Autodesk Inventor part; units mm, degrees
ref_plane "YZ Plane" through (0, 0, 0) normal (1, 0, 0) x (0, 1, 0)
ref_plane "XZ Plane" through (0, 0, 0) normal (0, 1, 0) x (-1, 0, 0)
ref_plane "XY Plane" through (0, 0, 0) normal (0, 0, 1) x (1, 0, 0)
sketch "Boceto1" plane through (0, 0, 0) normal (0, 1, 0) x (-1, 0, 0)
  circle A0 centre (0, 0) radius 0.99
  dimension "d0" = 1.98
extrude "Extrusión1" add sketch "Boceto1" along normal mid plane 4
sketch "Boceto2" plane through (0, 2, 0) normal (0, 1, 0) x (1, 0, 0)
  circle A0 centre (0, 0) radius 0.99
  circle A1 centre (0, 0) radius 2.7
  dimension "d3" = 5.4
extrude "Extrusión2" add sketch "Boceto2" along normal blind 0.5 contours A0 | A1
hole "Hole1" at (0, 2.5, 0) direction (0, -1, 0) diameter 1.96 end through all
hole "Hole2" at (0, 2.5, 0) direction (0, -1, 0) diameter 1.96 end through all countersink diameter 5.4 countersink angle 150
sketch "Boceto3" plane through (0, 2, 0) normal (0, -1, 0) x (1, 0, 0)
  line L0 (-1.55, 2.1185) -> (1.55, 2.1185)
  line L1 (1.55, 2.1185) -> (1.55, 10.6185)
  line L2 (1.55, 10.6185) -> (-1.55, 10.6185)
  line L3 (-1.55, 10.6185) -> (-1.55, 2.1185)
  line L4 (-1.55, 2.1185) -> (1.55, 10.6185) construction
  line L5 (1.55, 2.1185) -> (-1.55, 10.6185) construction
  point P0 (0, 6.3685)
  dimension "d24" = 3.1
  dimension "d25" = 8.5
extrude "Extrusión3" add sketch "Boceto3" against normal blind 0.5
hole "Hole3" at (0, 2.5, 0) direction (0, -1, 0) diameter 1.96 end through all countersink diameter 5.4 countersink angle 150
sketch "Boceto4" plane through (0, 2.5, 0) normal (0, 1, 0) x (1, 0, 0)
  line L0 (-1.55, -10.6185) -> (1.55, -10.6185)
  circle A0 centre (0, -10.6185) radius 1.55
  dimension "d39" = 3.1
extrude "Extrusión4" add sketch "Boceto4" against normal blind 0.5
properties part number "Conector"
Geometry: final body of the model. Coordinates: model frame, mm. Round coordinates to 2 decimals unless told otherwise and drop trailing zeros. Order: outer loops, then holes, each group sorted by start corner. A loop starts at its lowest first (then second) coordinate and runs counter-clockwise, first axis right, second up. Notation, with made-up numbers: (-13, 88.25) -> (23, 88.25) arc R21 ccw to (23, 125.25) -> close; hole circle Ø4 at (82.25, 81). An arc over 180 degrees is marked (long way). Use one line per item in the form item = value.
(1) First-contact query: pin 1 Ø1.5 at (x, z) = (-1, 10) entering from -Y; pin 2 Ø3 at (x, z) = (0, 0.5) entering from +Y; pin 3 Ø0.6 at (y, z) = (2, 6) entering from +X. Flat tips, straight axial feed; report the tip coordinate or a pass-through.
Results list:
pin_1 = 2
pin_2 = 2.31
pin_3 = 1.55
(2) Section D-D on z = 7.25. Return loops of the section in (x, y).
Results list:
outline = (-1.55, 2) -> (1.55, 2) -> (1.55, 2.5) -> (-1.55, 2.5) -> close
(3) Ray query, probe 1 along Y at (x, z) = (0.35, 10); probe 2 along X at (y, z) = (2.05, 2.5); probe 3 along Y at (x, z) = (-0.1, 2). Return the intervals inside material, ascending. Write a range as [from, to].
Results list:
probe_1 = [2, 2.5]
probe_2 = [-1.55, 1.55]
probe_3 = [2, 2.31]
(4) Section C-C on y = -0.55. Return loops of the section in (x, z), and give its area (3 significant figures).
Results list:
outline = circle Ø1.98 at (0, 0); hole circle Ø1.96 at (0, 0)
area = 0.0619 mm^2
